Verification items for the finished model (mm, model axes). Round coordinates to 2 decimals unless told otherwise and drop trailing zeros. Write each loop counter-clockwise with the first axis right and the second up, starting at its lowest first coordinate (ties: lowest second). Pieces come first, ordered by that corner, then holes. Notation, with made-up numbers: (16, 71) - (24, 71) arc R24 cw to (24, 101) - close; hole circle Ø4 at (-25.75, 6.25). An arc over 180 degrees is marked (long way). Write each question's results on one line, items separated by ' | '.
```python
from build123d import *

# Parameters (mm, degrees)
BOSS_EXTRUDE1_DEPTH = 52
SKETCH3_R           = 3.575
BOSS_EXTRUDE2_DEPTH = 2
FILLET2_R           = 2
HOLE1_D             = 3.2
HOLE1_CSINK_D       = 6.4
HOLE1_CSINK_ANGLE   = 90
HOLE2_D             = 3.2
HOLE3_D             = 3.2
HOLE3_CSINK_D       = 6.4
HOLE3_CSINK_ANGLE   = 90
FILLET1_R           = 3


with BuildPart() as part:
    # Sketch1 → Boss-Extrude1 (new body)
    with BuildSketch(Plane.XY):
        with BuildLine():
            ThreePointArc((14.981080915, 4.360756827), (0, -15.602851838), (-14.981080915, 4.360756827))
            Line((-14.981080915, 4.360756827), (-11.981080915, 4.360756827))
            ThreePointArc((-11.981080915, 4.360756827), (0, -12.75), (11.981080915, 4.360756827))
            Line((11.981080915, 4.360756827), (14.981080915, 4.360756827))
        make_face()
        with BuildLine():
            ThreePointArc((-15.543401376, 1.360756827), (-15.335775324, 2.874540085), (-14.981080915, 4.360756827))
            Line((-14.981080915, 4.360756827), (-24.981080915, 4.360756827))
            Line((-24.981080915, 4.360756827), (-24.981080915, 1.360756827))
            Line((-24.981080915, 1.360756827), (-15.543401376, 1.360756827))
        make_face()
        with BuildLine():
            Line((24.981080915, 4.360756827), (14.981080915, 4.360756827))
            ThreePointArc((14.981080915, 4.360756827), (15.335775324, 2.874540085), (15.543401376, 1.360756827))
            Line((15.543401376, 1.360756827), (24.981080915, 1.360756827))
            Line((24.981080915, 1.360756827), (24.981080915, 4.360756827))
        make_face()
    extrude(amount=-BOSS_EXTRUDE1_DEPTH)

    # Sketch3 → Boss-Extrude2 (add)
    with BuildSketch(Plane.XY):
        with BuildLine():
            Line((-3.809974466, 4.360756827), (-11.981080915, 4.360756827))
            ThreePointArc((-11.981080915, 4.360756827), (-12.749982881, -0.020893346), (-11.966724698, -4.4))
            Line((-11.966724698, -4.4), (11.966724698, -4.4))
            ThreePointArc((11.966724698, -4.4), (12.749982881, -0.020893346), (11.981080915, 4.360756827))
            Line((11.981080915, 4.360756827), (3.809974466, 4.360756827))
            ThreePointArc((3.809974466, 4.360756827), (0, 5.790691284), (-3.809974466, 4.360756827))
        make_face()
        Circle(SKETCH3_R, mode=Mode.SUBTRACT)
    extrude(amount=-BOSS_EXTRUDE2_DEPTH)

    # Fillet2
    fillet2_edges = [part.edges().sort_by_distance(p)[0] for p in [
        (-3.809974466, 4.360756827, -1),
        (3.809974466, 4.360756827, -1),
    ]]
    fillet(fillet2_edges, radius=FILLET2_R)

    # Hole1 (through all)
    with Locations(Plane(origin=(-8.5, -0.019621586, 0), x_dir=(1, 0, 0), z_dir=(0, 0, 1))):
        with Locations((0, 0), (17, 0)):
            CounterSinkHole(HOLE1_D / 2, HOLE1_CSINK_D / 2, counter_sink_angle=HOLE1_CSINK_ANGLE)

    # Hole2 (through all)
    with Locations(Plane(origin=(-20.981080915, 4.360756827, -35), x_dir=(1, 0, 0), z_dir=(0, 1, 0))):
        with Locations((0, 0), (0, -20), (41.96216183, -20), (41.96216183, 0)):
            Hole(HOLE2_D / 2)

    # Hole3 (through all)
    with Locations(Plane(origin=(-20.981080915, 4.360756827, -7), x_dir=(1, 0, 0), z_dir=(0, 1, 0))):
        with Locations((0, 0), (0, 38), (41.96216183, 38), (41.96216183, 0)):
            CounterSinkHole(HOLE3_D / 2, HOLE3_CSINK_D / 2, counter_sink_angle=HOLE3_CSINK_ANGLE)

    # Fillet1
    fillet1_edges = [part.edges().sort_by_distance(p)[0] for p in [
        (11.966724698, -4.4, -1),
        (-11.966724698, -4.4, -1),
    ]]
    fillet(fillet1_edges, radius=FILLET1_R)


solid = part.part
```
(1) Section check A-A (x = 0). Record the cut outline in (y, z) (3 decimals).
Answer:
outline: (-15.603, -52) - (-12.75, -52) - (-12.75, 0) - (-15.603, 0) - close; (-4.4, -2) - (-3.575, -2) - (-3.575, 0) - (-4.4, 0) - close; (3.575, -2) - (5.791, -2) - (5.791, 0) - (3.575, 0) - close
(2) Mould release check, pull along Y, two halves, no side actions. Record for faces 1 (the cylindrical face through (-0.343, -12.745, -25.636)), 2 (the flat face through (17, 4.361, -26)), 3 (the flat face through (-24.981, 3, -26)): released by +Y, released by -Y, zero draft, split by the parting line, or undercut.
Answer:
face 1: undercut | face 2: released by +Y | face 3: zero draft
(3) Go/stop test with flat-tipped pins: pin 1 Ø1.9 at (x, z) = (-20.98, -15) entering from -Y; pin 2 Ø6 at (x, z) = (17, -31) entering from +Y; pin 3 Ø3.5 at (x, z) = (20.98, -7) entering from +Y; pin 4 Ø2 at (y, z) = (-4, -25) entering from -X. Record where each tip stops, or that it passes through.
Answer:
pin 1: through | pin 2: y = 4.36 | pin 3: y = 2.91 | pin 4: x = -15.31
(4) Thickness scan on L1, parallel to X at y = 0.25, z = -34; L2, parallel to X at y = 3.75, z = -7.5; L3, parallel to X at y = 2.5, z = -24. Record the ranges inside material, lowest first.
Answer:
L1: -15.6 to -12.75, 12.75 to 15.6 | L2: -24.98 to -23.52, -18.44 to -12.19, 12.19 to 18.44, 23.52 to 24.98 | L3: -24.98 to -12.5, 12.5 to 24.98
(5) Section check C-C (z = -7). Record the cut outline in (x, y).
Answer:
outline: (-24.98, 1.36) - (-22.58, 1.36) - (-22.58, 2.76) - (-24.18, 4.36) - (-24.98, 4.36) - close; (-19.38, 1.36) - (-15.54, 1.36) arc R15.6 ccw (long way) to (15.54, 1.36) - (19.38, 1.36) - (19.38, 2.76) - (17.78, 4.36) - (11.98, 4.36) arc R12.75 cw (long way) to (-11.98, 4.36) - (-17.78, 4.36) - (-19.38, 2.76) - close; (22.58, 1.36) - (24.98, 1.36) - (24.98, 4.36) - (24.18, 4.36) - (22.58, 2.76) - close
(6) Section check B-B (z = -35). Record the cut outline in (x, y).
Answer:
outline: (-24.98, 1.36) - (-22.58, 1.36) - (-22.58, 4.36) - (-24.98, 4.36) - close; (-19.38, 1.36) - (-15.54, 1.36) arc R15.6 ccw (long way) to (15.54, 1.36) - (19.38, 1.36) - (19.38, 4.36) - (11.98, 4.36) arc R12.75 cw (long way) to (-11.98, 4.36) - (-19.38, 4.36) - close; (22.58, 1.36) - (24.98, 1.36) - (24.98, 4.36) - (22.58, 4.36) - close
